Job drawing, mm, ordinate dimensions from the low corner. One solid piece. Round coordinates to 2 decimals unless told otherwise and drop trailing zeros. Loops run counter-clockwise (first coordinate to the right, second up) from the corner with the lowest first, then second, coordinate; pieces in that order, holes last.
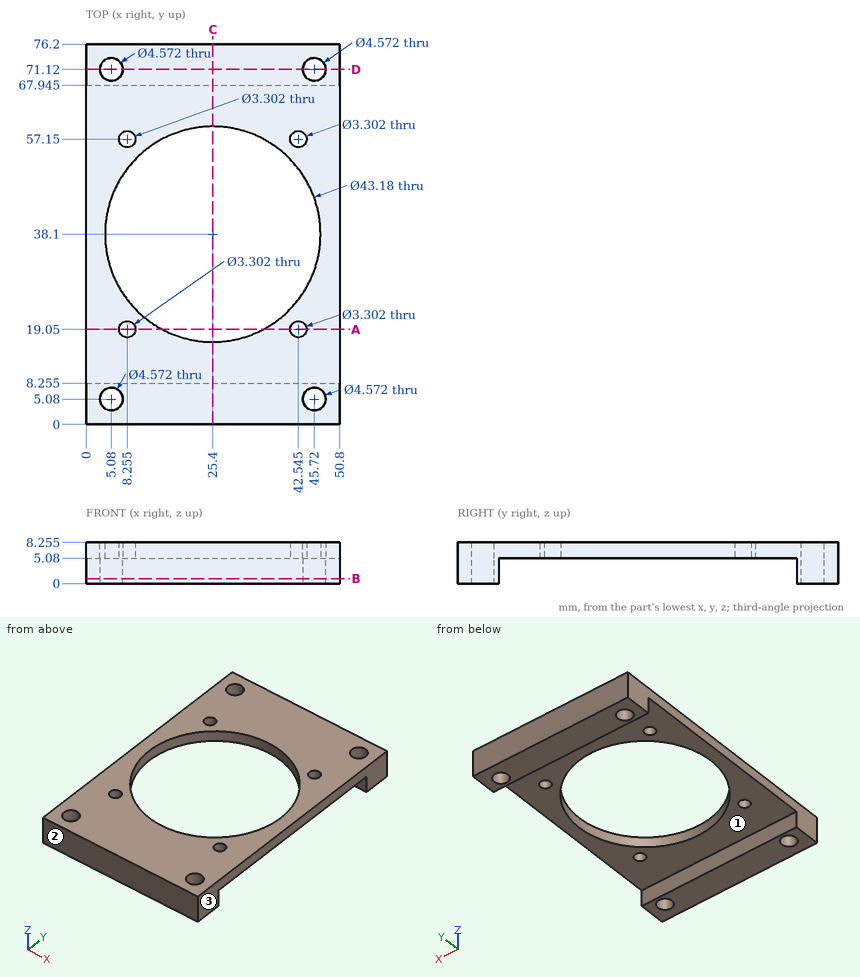
(1) Slice it at A-A on y = 19.05. List the corners of the cut face in (x, z) (3 decimals).
Responses:
outline: (0, 5.08) - (6.604, 5.08) - (6.604, 8.255) - (0, 8.255) - close; (9.906, 5.08) - (15.24, 5.08) - (15.24, 8.255) - (9.906, 8.255) - close; (35.56, 5.08) - (40.894, 5.08) - (40.894, 8.255) - (35.56, 8.255) - close; (44.196, 5.08) - (50.8, 5.08) - (50.8, 8.255) - (44.196, 8.255) - close
(2) Slice it at D-D on y = 71.12. List the corners of the cut face in (x, z) (3 decimals), plus the area to 3 significant figures.
Responses:
outline: (0, 0) - (2.794, 0) - (2.794, 8.255) - (0, 8.255) - close; (7.366, 0) - (43.434, 0) - (43.434, 8.255) - (7.366, 8.255) - close; (48.006, 0) - (50.8, 0) - (50.8, 8.255) - (48.006, 8.255) - close
area: 344 mm2
(3) Pull direction Y, two halves, no side cores. Call the marked faces 1, 2 and 3: +Y half, -Y half, draft (parallel to the pull), parting line (faces both ways), or undercut.
Responses:
face 1: undercut
face 2: -Y half
face 3: draft
(4) Pin check, flat tips, straight feed: P1, Ø5.5, axis at x = 8.255, y = 19.05, coming from the -Z side; P2, Ø3.5, axis at x = 5.08, y = 5.08, coming from the +Z side. Stop position of each tip, or through.
Responses:
P1: stops at z = 5.08
P2: passes through
(5) Probe line 1 (Y direction, x = 5.08, z = 2.75) (3 decimals); line 2 (Y direction, x = 46, z = 1.5) (3 decimals); line 3 (Y direction, x = 29.5, z = 0.75) (3 decimals). List the from-to ranges inside material, lowest first.
Responses:
line 1: y = 0 to 2.794, 7.366 to 8.255, 67.945 to 68.834, 73.406 to 76.2
line 2: y = 0 to 2.811, 7.349 to 8.255, 67.945 to 68.851, 73.389 to 76.2
line 3: y = 0 to 8.255, 67.945 to 76.2
(6) Slice it at B-B on z = 1. List the corners of the cut face in (x, y) (3 decimals), plus the area to 3 significant figures.
Responses:
outline: (0, 0) - (50.8, 0) - (50.8, 8.255) - (0, 8.255) - close; (0, 67.945) - (50.8, 67.945) - (50.8, 76.2) - (0, 76.2) - close; hole circle Ø4.572 at (5.08, 5.08); hole circle Ø4.572 at (5.08, 71.12); hole circle Ø4.572 at (45.72, 5.08); hole circle Ø4.572 at (45.72, 71.12)
area: 773 mm2
(7) Slice it at C-C on x = 25.4. List the corners of the cut face in (y, z) (3 decimals), plus the area to 3 significant figures.
Responses:
outline: (0, 0) - (8.255, 0) - (8.255, 5.08) - (16.51, 5.08) - (16.51, 8.255) - (0, 8.255) - close; (59.69, 5.08) - (67.945, 5.08) - (67.945, 0) - (76.2, 0) - (76.2, 8.255) - (59.69, 8.255) - close
area: 189 mm2
